```python
from build123d import *

# Parameters (mm, degrees)
SKETCH1_W           = 117
SKETCH1_H           = 55.6
BOSS_EXTRUDE1_DEPTH = 16.3
SKETCH2_W           = 79
SKETCH2_H           = 23
BOSS_EXTRUDE2_DEPTH = 13.5
SKETCH4_W           = 11.183333333
SKETCH4_H           = 19.4
SKETCH4_W_2         = 11.183333334
CUT_EXTRUDE2_DEPTH  = 13.5
CUT_EXTRUDE1_DEPTH  = 79
BOSS_EXTRUDE3_DEPTH = 50.6
SKETCH7_R           = 2.5
CUT_EXTRUDE3_DEPTH  = 3.35
FILLET1_R           = 0.5


with BuildPart() as part:
    # Sketch1 → Boss-Extrude1 (new body)
    with BuildSketch(Plane(origin=(0, 0, 0), x_dir=(1, 0, 0), z_dir=(0, 1, 0))):
        Rectangle(SKETCH1_W, SKETCH1_H)
    extrude(amount=BOSS_EXTRUDE1_DEPTH)

    # Sketch2 → Boss-Extrude2 (add)
    with BuildSketch(Plane(origin=(0, 16.3, 0), x_dir=(1, 0, 0), z_dir=(0, 1, 0))):
        with Locations((0, -16.3)):
            Rectangle(SKETCH2_W, SKETCH2_H)
    extrude(amount=BOSS_EXTRUDE2_DEPTH)

    # Sketch4 → Cut-Extrude2 (cut)
    with BuildSketch(Plane(origin=(0, 29.8, 0), x_dir=(1, 0, 0), z_dir=(0, 1, 0))):
        with Locations((-32.208333334, -18.1)):
            Rectangle(SKETCH4_W, SKETCH4_H)
        with Locations((-19.325, -18.1)):
            Rectangle(SKETCH4_W_2, SKETCH4_H)
        with Locations((-6.441666667, -18.1)):
            Rectangle(SKETCH4_W, SKETCH4_H)
        with Locations((6.441666667, -18.1)):
            Rectangle(SKETCH4_W, SKETCH4_H)
        with Locations((19.325, -18.1)):
            Rectangle(SKETCH4_W_2, SKETCH4_H)
        with Locations((32.208333334, -18.1)):
            Rectangle(SKETCH4_W, SKETCH4_H)
    extrude(amount=-CUT_EXTRUDE2_DEPTH, mode=Mode.SUBTRACT)

    # Sketch3 → Cut-Extrude1 (cut)
    with BuildSketch(Plane(origin=(39.5, 0, 0), x_dir=(0, 0, -1), z_dir=(1, 0, 0))):
        with BuildLine():
            Line((-27.8, 16.3), (-25.3, 16.3))
            Line((-25.3, 16.3), (-25.3, 25.55))
            ThreePointArc((-25.3, 25.55), (-24.05520382, 28.55520382), (-21.05, 29.8))
            Line((-21.05, 29.8), (-27.8, 29.8))
            Line((-27.8, 29.8), (-27.8, 16.3))
        make_face()
        Polygon((-9.9, 29.8), (-8.4, 28.3), (-4.8, 28.3), (-4.8, 29.8), align=None)
    extrude(amount=-CUT_EXTRUDE1_DEPTH, mode=Mode.SUBTRACT)

    # Sketch5 → Boss-Extrude3 (add)
    with BuildSketch(Plane.XY.offset(25.3)):
        Polygon((-58.5, 7.655574629), (-63.7, -2.55), (-76.25, -2.55), (-76.25, -4.9), (-57.82, -4.9), (-57.82, -2.5), (-54.17, -2.5), (-54.17, -4.9), (-52.17, -4.9), (-52.17, -2.5), (-48.52, -2.5), (-48.52, -4.9), (-46.52, -4.9), (-46.52, 0), (-58.5, 0), align=None)
        Polygon((58.5, 0), (58.5, 7.655574629), (63.7, -2.55), (76.25, -2.55), (76.25, -4.9), (57.82, -4.9), (57.82, -2.5), (54.17, -2.5), (54.17, -4.9), (52.17, -4.9), (52.17, -2.5), (48.52, -2.5), (48.52, -4.9), (46.52, -4.9), (46.52, 0), align=None)
    extrude(amount=-BOSS_EXTRUDE3_DEPTH)

    # Sketch7 → Cut-Extrude3 (cut, through all)
    with BuildSketch(Plane(origin=(0, -2.55, 0), x_dir=(1, 0, 0), z_dir=(0, 1, 0))):
        with Locations((-69.975, 12.8)):
            Circle(SKETCH7_R)
        with Locations((69.975, 12.8)):
            Circle(SKETCH7_R)
        with Locations((69.975, -12.8)):
            Circle(SKETCH7_R)
        with Locations((-69.975, -12.8)):
            Circle(SKETCH7_R)
    extrude(amount=-CUT_EXTRUDE3_DEPTH, mode=Mode.SUBTRACT)

    # Fillet1
    fillet1_edges = [part.edges().sort_by_distance(p)[0] for p in [
        (-46.52, -4.9, 0),
        (-48.52, -4.9, 0),
        (-48.52, -2.5, 0),
        (-52.17, -2.5, 0),
        (-52.17, -4.9, 0),
        (-54.17, -4.9, 0),
        (-54.17, -2.5, 0),
        (-57.82, -2.5, 0),
        (-57.82, -4.9, 0),
        (-76.25, -4.9, 0),
        (-76.25, -2.55, 0),
        (-63.7, -2.55, 0),
        (63.7, -2.55, 0),
        (76.25, -2.55, 0),
        (76.25, -4.9, 0),
        (57.82, -4.9, 0),
        (57.82, -2.5, 0),
        (54.17, -2.5, 0),
        (54.17, -4.9, 0),
        (52.17, -4.9, 0),
        (52.17, -2.5, 0),
        (48.52, -2.5, 0),
        (48.52, -4.9, 0),
        (46.52, -4.9, 0),
    ]]
    fillet(fillet1_edges, radius=FILLET1_R)


solid = part.part
```
Input: part model. Units: mm. Frame: model coordinates. A direction names the side the tool comes from. Round coordinates to 2 decimals unless told otherwise and drop trailing zeros. Loops run counter-clockwise (first coordinate to the right, second up) from the corner with the lowest first, then second, coordinate; pieces in that order, holes last. Notation, with made-up numbers: (81.25, 13.5) -> (138.25, 13.5) arc R33 ccw to (138.25, 49.5) -> close; hole circle Ø8 at (86.25, -16). An arc over 180 degrees is marked (long way). One line per item, written item: value.
(1) Material intervals for line 1 (Y direction, x = -54.5, z = -19); line 2 (Z direction, x = -21, y = 22); line 3 (Y direction, x = -53, z = 21.5), sorted ascending. Write a range as [from, to].
Geometry check:
line 1: [-2.53, 16.3]
line 2: [4.8, 8.4]
line 3: [-4.9, 16.3]
(2) Section A-A (x = -23.5). Return the cut outline in (y, z).
Geometry check:
outline: (0, -27.8) -> (16.3, -27.8) -> (16.3, 4.8) -> (28.3, 4.8) -> (28.3, 8.4) -> (16.3, 8.4) -> (16.3, 27.8) -> (0, 27.8) -> close
(3) Pin query (flat end, axial travel): pin 1 (4 mm diameter, centred on x = -66.5, y = -1, fed in from -Z); pin 2 (1 mm diameter, centred on x = -45.5, z = -11.5, fed in from +Y); pin 3 (5.5 mm diameter, centred on x = -33.5, y = 21.5, fed in from +Z). Return the tip coordinate at first contact, or that it passes through.
Geometry check:
pin 1: z = -25.3
pin 2: y = 16.3
pin 3: z = 8.4
(4) Section B-B (z = 12.8). Give the number of separate pieces and of enclosed holes in the cut face, plus the area to 3 significant figures.
Geometry check:
separate pieces: 3
enclosed holes: 0
area: 2,260 mm2
(5) Section C-C (y = 10.5). Return the cut outline in (x, z).
Geometry check:
outline: (-58.5, -27.8) -> (58.5, -27.8) -> (58.5, 27.8) -> (-58.5, 27.8) -> close
(6) Mould query, pull axis X, two halves, no side actions, for faces 6 (the face through (-37.8, 23, 17)), 7 (the face through (-12.87, 28.52, 24.09)). Classes: pulls with the +X half, pulls with the -X half, needs draft (parallel to the pull), parting line crosses it, or undercut.
Geometry check:
face 6: undercut
face 7: needs draft
(7) Set-up query: faces 1 (the face through (1, 28.3, 7)), 2 (the face through (-7, 22, 8.4)), 3 (the face through (56, -2.5, 0)), 4 (the face through (70, -2.55, 0)), 5 (the face through (67, -4.9, 0)). Return all of +Z, -Z, +X, -X, +Y, -Y with unobstructed straight access to the full face (end or side cutting, diameter ignored); none if empty.
Geometry check:
face 1: -Z, +X, -X, +Y
face 2: +Z, +Y
face 3: +Z, -Z, -Y
face 4: +Z, -Z, +X, +Y
face 5: +Z, -Z, +X, -X, -Y
